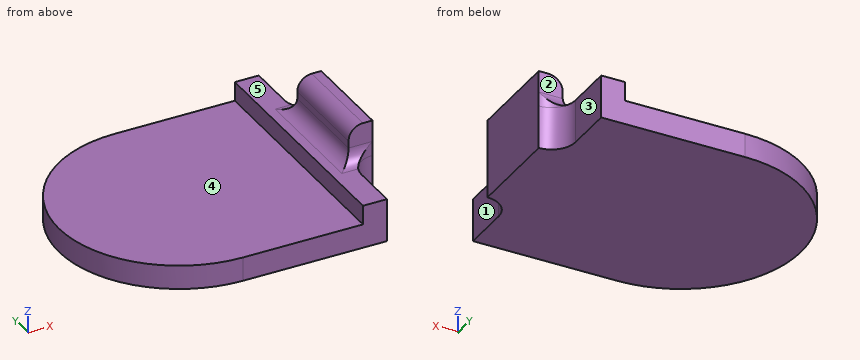
```python
from build123d import *

# Parameters (mm, degrees)
F1_DEPTH     = 5
F2_W         = 5
F2_H         = 50
F3_DEPTH     = 4
F4_W         = 5
F4_H         = 20
F5_DEPTH     = 11.5
F6_T1_DEPTH  = 9
F7_T1_DEPTH  = 20
F7_T6_DEPTH  = 5
F7_S7_R      = 5.0000000001
F7_T8_DEPTH  = 5
F7_T12_DEPTH = 5
F7_S13_R     = 5.0000000001
F7_T14_DEPTH = 5
F7_T19_DEPTH = 12.5
F7_T24_DEPTH = 27.5
F7_T31_DEPTH = 27.5
F7_T35_DEPTH = 12.5
F7_T39_DEPTH = 35


# Not quite as in the source:
# - a fillet or chamfer that OpenCascade refuses, or shapes differently, is made with other operations: its cross-section is extruded or revolved along the edge and cut away or added


with BuildPart() as f1:
    # F0 (on Top) → F1 (new body)
    with BuildSketch(Plane.XY):
        with BuildLine():
            Line((30, 25), (0, 25))
            ThreePointArc((0, 25), (-25, 0), (0, -25))
            Line((0, -25), (30, -25))
            Line((30, -25), (30, -10))
            Line((30, -10), (35, -10))
            Line((35, -10), (35, 10))
            Line((35, 10), (30, 10))
            Line((30, 10), (30, 25))
        make_face()
    extrude(amount=F1_DEPTH)

    # F2 (on face) → F3 (join)
    with BuildSketch(Plane.XY.offset(5)):
        with Locations((27.5, 0)):
            Rectangle(F2_W, F2_H)
    extrude(amount=F3_DEPTH)

    # F4 (on face) → F5 (join)
    with BuildSketch(Plane.XY.offset(5)):
        with Locations((32.5, 0)):
            Rectangle(F4_W, F4_H)
    extrude(amount=F5_DEPTH)

    # F6: fillet of radius 5 on 3 edges, made by hand

    # F6_s2 → F6_t1 (join)
    with BuildSketch(Plane.XY):
        with BuildLine():
            ThreePointArc((30, -15), (31.4644660941, -11.4644660941), (35, -10))
            Line((35, -10), (30, -10))
            Line((30, -10), (30, -15))
        make_face()
        with BuildLine():
            ThreePointArc((30, 15), (31.4644660941, 11.4644660941), (35, 10))
            Line((35, 10), (30, 10))
            Line((30, 10), (30, 15))
        make_face()
    extrude(amount=F6_T1_DEPTH)

    # F7: fillet of radius 3 on 4 edges, made by hand

    # F7_s2 → F7_t1 (join)
    with BuildSketch(Plane.XZ.offset(-10)):
        with BuildLine():
            ThreePointArc((27, 9), (29.1213203436, 9.8786796564), (30, 12))
            Line((30, 12), (30, 9))
            Line((30, 9), (27, 9))
        make_face()
    extrude(amount=F7_T1_DEPTH)


with BuildPart() as f7_tool4:
    # F7_s5 → F7_t6 (new body)
    with BuildSketch(Plane.YZ.offset(35)):
        with BuildLine():
            ThreePointArc((-13, 9), (-10.8786796564, 9.8786796564), (-10, 12))
            Line((-10, 12), (-10, 9))
            Line((-10, 9), (-13, 9))
        make_face()
    extrude(amount=-F7_T6_DEPTH)

    # F7_s7 → F7_t8 (cut, symmetric)
    with BuildSketch(Plane.XY.offset(10.5)):
        with Locations((35.0000000001, -15.0000000001)):
            Circle(F7_S7_R)
    extrude(amount=F7_T8_DEPTH, both=True, mode=Mode.SUBTRACT)


with BuildPart() as f1_1:
    add(f1.part)

    # F7_t3: union F7_tool4
    add(f7_tool4.part)


with BuildPart() as f7_tool10:
    # F7_s11 → F7_t12 (new body)
    with BuildSketch(Plane.YZ.offset(35)):
        with BuildLine():
            ThreePointArc((13, 9), (10.8786796564, 9.8786796564), (10, 12))
            Line((10, 12), (10, 9))
            Line((10, 9), (13, 9))
        make_face()
    extrude(amount=-F7_T12_DEPTH)

    # F7_s13 → F7_t14 (cut, symmetric)
    with BuildSketch(Plane.XY.offset(10.5)):
        with Locations((35.0000000001, 15.0000000001)):
            Circle(F7_S13_R)
    extrude(amount=F7_T14_DEPTH, both=True, mode=Mode.SUBTRACT)


with BuildPart() as f1_2:
    add(f1_1.part)

    # F7_t9: union F7_tool10
    add(f7_tool10.part)


with BuildPart() as f7_tool17:
    # F7_s18 → F7_t19 (new body)
    with BuildSketch(Plane.YZ.offset(35)):
        with BuildLine():
            ThreePointArc((-13, 9), (-10.8786796564, 9.8786796564), (-10, 12))
            Line((-10, 12), (-10, 9))
            Line((-10, 9), (-13, 9))
        make_face()
    extrude(amount=-F7_T19_DEPTH)

    split(bisect_by=Plane.YZ.offset(25), keep=Keep.TOP)

    split(bisect_by=Plane.YZ.offset(30), keep=Keep.BOTTOM)


with BuildPart() as f7_tool22:
    # F7_s23 → F7_t24 (new body)
    with BuildSketch(Plane.XZ.offset(17.5)):
        with BuildLine():
            ThreePointArc((27, 9), (29.1213203436, 9.8786796564), (30, 12))
            Line((30, 12), (30, 9))
            Line((30, 9), (27, 9))
        make_face()
    extrude(amount=-F7_T24_DEPTH)

    split(bisect_by=Plane.XZ.offset(10), keep=Keep.TOP)


with BuildPart() as f7_tool17_1:
    add(f7_tool17.part)

    # F7_t26: intersect F7_tool22
    add(f7_tool22.part, mode=Mode.INTERSECT)


with BuildPart() as f1_3:
    add(f1_2.part)

    # F7_t15: union F7_tool17
    add(f7_tool17_1.part)


with BuildPart() as f7_tool29:
    # F7_s30 → F7_t31 (new body)
    with BuildSketch(Plane.XZ.offset(10)):
        with BuildLine():
            ThreePointArc((27, 9), (29.1213203436, 9.8786796564), (30, 12))
            Line((30, 12), (30, 9))
            Line((30, 9), (27, 9))
        make_face()
    extrude(amount=-F7_T31_DEPTH)

    split(bisect_by=Plane.XZ.offset(-10), keep=Keep.BOTTOM)


with BuildPart() as f7_tool33:
    # F7_s34 → F7_t35 (new body)
    with BuildSketch(Plane.YZ.offset(35)):
        with BuildLine():
            ThreePointArc((13, 9), (10.8786796564, 9.8786796564), (10, 12))
            Line((10, 12), (10, 9))
            Line((10, 9), (13, 9))
        make_face()
    extrude(amount=-F7_T35_DEPTH)

    split(bisect_by=Plane.YZ.offset(25), keep=Keep.TOP)

    split(bisect_by=Plane.YZ.offset(30), keep=Keep.BOTTOM)


with BuildPart() as f7_tool29_1:
    add(f7_tool29.part)

    # F7_t38: intersect F7_tool33
    add(f7_tool33.part, mode=Mode.INTERSECT)


with BuildPart() as f1_4:
    add(f1_3.part)

    # F7_t27: union F7_tool29
    add(f7_tool29_1.part)

    # F7_s40 → F7_t39 (cut)
    with BuildSketch(Plane.XZ.offset(-17.5)):
        with BuildLine():
            ThreePointArc((30, 13.5), (30.8786796564, 15.6213203436), (33, 16.5))
            Line((33, 16.5), (30, 16.5))
            Line((30, 16.5), (30, 13.5))
        make_face()
    extrude(amount=F7_T39_DEPTH, mode=Mode.SUBTRACT)


solid = f1_4.part
```
Design review of the part built by this model. Coordinates are the model's own, in mm. Face numbers are marked on the shaded views. A direction names the side the tool comes from. Round coordinates to 2 decimals unless told otherwise and drop trailing zeros. Write each loop counter-clockwise with the first axis right and the second up, starting at its lowest first coordinate (ties: lowest second). Pieces come first, ordered by that corner, then holes. Notation, with made-up numbers: (40, -9) -> (61, -9) arc R37 cw to (61, 29) -> close; hole circle Ø5 at (50, -1.75). An arc over 180 degrees is marked (long way). Write item = value, one per line. Start each with the question number.
1) Wall thickness on probe 1 along X at (y, z) = (4, 13.25); probe 2 along Z at (x, y) = (9, -17); probe 3 along X at (y, z) = (-7.5, 7.25): over which ranges is each line inside the solid? List them lowest first. Write a range as from..to.
2) Clearance check with flat-ended pins moving along their axes: pin 1 (2 mm diameter, centred on y = 9, z = 7.5, fed in from -X); pin 2 (12 mm diameter, centred on x = -15, y = -14.5, fed in from +Z); pin 3 (1.6 mm diameter, centred on x = 28.5, y = -7.5, fed in from +Z). State where each tip first meets the part, or that it passes through.
3) Take a section at A-A, the plane y = 0. State the section outline as (x, z) points.
4) Take a section at C-C, the plane x = 26. State the section outline as (y, z) points.
5) Take a section at B-B, the plane z = 1.5. State the section outline as (x, y) points, plus the area to 3 significant figures.
6) Tool access review of the marked faces 1, 2, 3, 4 and 5: name each direction out of +Z, -Z, +X, -X, +Y, -Y from which nothing blocks a thin tool from reaching the whole face with its end or side.
7) Take a section at D-D, the plane z = 7.25. State the section outline as (x, y) points, plus the area to 3 significant figures.
Results list:
q1.probe_1 = 30..35
q1.probe_2 = 0..5
q1.probe_3 = 25..35
q2.pin_1 = 25
q2.pin_2 = 5
q2.pin_3 = 10.07
q3.outline = (-25, 0) -> (35, 0) -> (35, 16.5) -> (33, 16.5) arc R3 ccw to (30, 13.5) -> (30, 12) arc R3 cw to (27, 9) -> (25, 9) -> (25, 5) -> (-25, 5) -> close
q4.outline = (-25, 0) -> (25, 0) -> (25, 9) -> (-25, 9) -> close
q5.outline = (0, -25) -> (30, -25) -> (30, -15) arc R5 cw to (35, -10) -> (35, 10) arc R5 cw to (30, 15) -> (30, 25) -> (0, 25) arc R25 ccw to start
q5.area = 2,590 mm²
q6.face_1 = +Z, -Z, +X, -Y
q6.face_2 = +Z, +X, -X, +Y
q6.face_3 = +Z, -Z, +X, +Y
q6.face_4 = +Z, -X, +Y, -Y
q6.face_5 = +Z, -X
q7.outline = (25, -25) -> (30, -25) -> (30, -15) arc R5 cw to (35, -10) -> (35, 10) arc R5 cw to (30, 15) -> (30, 25) -> (25, 25) -> close
q7.area = 361 mm²
